from build123d import *

# Parameters (mm, degrees)
F0_R      = 43.6
F2_R      = 44.6
F4_R      = 50.1
F4_R_2    = 44.6
F5_DEPTH  = 4
F13_DEPTH = 8.5
F14_R     = 3.25
F15_DEPTH = 5


with BuildPart() as f3:
    # F0 (on Top) → F3 section 0
    with BuildSketch(Plane.XY):
        Circle(F0_R)
    # F2 (on offset) → F3 section 1
    with BuildSketch(Plane.XY.offset(-17.2)):
        Circle(F2_R)
    loft()

    # F4 (on face) → F5 (join)
    with BuildSketch(Plane(origin=(0, 0, -17.2), x_dir=(1, 0, 0), z_dir=(0, 0, -1))):
        Circle(F4_R)
        Circle(F4_R_2, mode=Mode.SUBTRACT)
        Circle(F4_R_2)
    extrude(amount=F5_DEPTH)

    # F6 (on Front) → F7 (revolve)
    with BuildSketch(Plane.XZ):
        with BuildLine():
            Line((-43.6, 0), (0, 0))
            Line((0, 0), (0, 12.5))
            ThreePointArc((0, 12.5), (-22.6782384677, 9.3132957755), (-43.6, 0))
        make_face()
    revolve(axis=Axis((0, 0, 11.7095857859), (0, 0, 1)))

    # F9 (on offset) → F10 (join, up to the next surface of F3)
    with BuildSketch(Plane.XY.offset(14)):
        with BuildLine():
            ThreePointArc((43.6, 0), (43.4872818741, 3.1330999347), (43.1497103119, 6.25))
            Line((43.1497103119, 6.25), (-43.1497103119, 6.25))
            ThreePointArc((-43.1497103119, 6.25), (-43.6, 0), (-43.1497103119, -6.25))
            Line((-43.1497103119, -6.25), (43.1497103119, -6.25))
            ThreePointArc((43.1497103119, -6.25), (43.4872818741, -3.1330999347), (43.6, 0))
        make_face()
    extrude(until=Until.NEXT, dir=(0, 0, -1))

    # F12 (on offset) → F13 (join)
    with BuildSketch(Plane.XZ.offset(43.6)):
        Polygon((2.8867513459, -13.6), (5.7735026919, -8.6), (2.8867513459, -3.6), (-2.8867513459, -3.6), (-5.7735026919, -8.6), (-2.8867513459, -13.6), align=None)
    extrude(amount=F13_DEPTH)

    # F14 (on face) → F15 (cut)
    with BuildSketch(Plane.XZ.offset(52.1)):
        with Locations((0, -8.6)):
            Circle(F14_R)
    extrude(amount=-F15_DEPTH, mode=Mode.SUBTRACT)


solid = f3.part
Part model, mm, in its own coordinate system. A direction names the side the tool comes from. Coordinates: 2 decimals unless noted, no trailing zeros. Loops run counter-clockwise (first coordinate to the right, second up) from the corner with the lowest first, then second, coordinate; pieces in that order, holes last. Notation, with made-up numbers: (81, 68.25) - (113, 68.25) arc R29 ccw to (113, 107.25) - close; hole circle Ø9 at (-22, 28). An arc over 180 degrees is marked (long way). Write each question's results on one line, items separated by ' | '. Start each with the question number.
Q1. Slice it at C-C on z = -7. Give the cut face in (x, y), and give its area (3 significant figures).
Q2. Two-plate mould, pull along Z, no slides. Class faces 1 (the cylindrical face through (-0.423, -49.635, -5.378)), 2 (the cylindrical face through (-43.6, 0.1, 7.1)), 3 (the flat face through (-4.31, -47.848, -6.065)): +Z half, -Z half, draft (parallel to the pull), parting line (faces both ways), or undercut.
Q3. Slice it at B-B on z = 5. Give the cut face in (x, y).
Q4. Which spindle directions (+Z, -Z, +X, -X, +Y, -Y) get a long thin tool onto all of the face, cutting with end or side? Do faces 4 (the flat face through (0, -47.1, -9)), 5 (the flat face through (1, 6.25, 13)), 6 (the flat face through (4.31, -47.852, -11.135)), 7 (the flat face through (-1, -6.25, 13)), 8 (the flat face through (4.35, -47.848, -6.135)). Say none if no direction does.
Q5. Drop flat-ended pins along their axis: pin 1 Ø5 at (x, z) = (1.5, -8.5) entering from -Y; pin 2 Ø12 at (y, z) = (-22.5, 8.5) entering from -X; pin 3 Ø6.5 at (x, y) = (0.5, -49) entering from +Z; pin 4 Ø1 at (y, z) = (-23.5, -1) entering from -X. Give the stop position or say it passes through.
Q6. Slice it at A-A on x = 0. Give the cut face in (y, z).
Q7. Probe line 1 along Z through (x, y) = (0, -49.5); line 2 along Y through (x, z) = (-35, 12); line 3 along Y through (x, z) = (16, -11.5). List the from-to ranges inside material, lowest first.
Answer:
1) outline: (-4.85, -52.1) - (-2.83, -52.1) - (-2.83, -47.1) - (2.83, -47.1) - (2.83, -52.1) - (4.85, -52.1) - (4.85, -43.74) arc R44.01 ccw (long way) to (-4.85, -43.74) - close | area: 6,140 mm2
2) face 1: undercut | face 2: draft | face 3: +Z half
3) outline: (-43.15, -6.25) - (-33.75, -6.25) arc R34.32 ccw to (33.75, -6.25) - (43.15, -6.25) arc R43.6 ccw to (43.15, 6.25) - (33.75, 6.25) arc R34.32 ccw to (-33.75, 6.25) - (-43.15, 6.25) arc R43.6 ccw to start
4) face 4: -Y | face 5: +Z, +Y | face 6: +X, -Y | face 7: +Z, -Y | face 8: +Z, +X, -Y
5) pin 1: stops at y = -52.1 | pin 2: stops at x = -32.83 | pin 3: stops at z = -3.6 | pin 4: stops at x = -37.11
6) outline: (-52.1, -13.6) - (-44.39, -13.6) - (-44.6, -17.2) - (-50.1, -17.2) - (-50.1, -21.2) - (50.1, -21.2) - (50.1, -17.2) - (44.6, -17.2) - (43.6, 0) arc R82.29 ccw to (6.25, 12.26) - (6.25, 14) - (-6.25, 14) - (-6.25, 12.26) arc R82.29 ccw to (-43.6, 0) - (-43.81, -3.6) - (-52.1, -3.6) - (-52.1, -5.35) - (-47.1, -5.35) - (-47.1, -11.85) - (-52.1, -11.85) - close
7) line 1: z = -21.2 to -17.2, -13.6 to -11.85, -5.35 to -3.6 | line 2: y = -6.25 to 6.25 | line 3: y = -41.28 to 41.28
